Answer from the drawing. Dimensions are ordinates in mm from the lowest x, y and z of the part. A direction names the side the tool comes from. Coordinates: 2 decimals unless noted, no trailing zeros. Order: outer loops, then holes, each group sorted by start corner. A loop starts at its lowest first (then second) coordinate and runs counter-clockwise, first axis right, second up. Notation, with made-up numbers: (15, 7.25) -> (51, 7.25) arc R27 ccw to (51, 25.25) -> close; hole circle Ø5 at (19.25, -1). An arc over 180 degrees is marked (long way). Answer as a JSON object with one key per item and string values. Group by question number.
1) A tool of negligible diameter and unlimited length cuts with its end or side. For the marked faces 1 and 2, from which of +Z, -Z, +X, -X, +Y, -Y can it reach the whole face along a straight path? Write none if from no direction.
2) Given pin 1 (10.5 mm diameter, centred on x = 39.5, y = 15, fed in from -Z), flat-ended and moving along its own axis, determine where the tip first touches the part or whether it passes through.
3) Section C-C on z = 11.75 is taken. Determine the outline of the cut face in (x, y), and give its area (3 significant figures).
4) Determine the mould class of the marked faces 3, 4 and 5 for opening direction Y: released by +Y, released by -Y, zero draft, split by the parting line, or undercut.
5) Section A-A on y = 15 is taken. Count the separate pieces of the cut face and the enclosed holes in it, and give its area (3 significant figures).
6) Consider L1, parallel to Y at x = 8.5, z = 15; L2, parallel to Y at x = 42, z = 15; L3, parallel to X at y = 13.25, z = 8.5. Determine where each line is inside the solid, lowest interval first.
7) Section B-B on x = 8.5 is taken. Determine the outline of the cut face in (y, z).
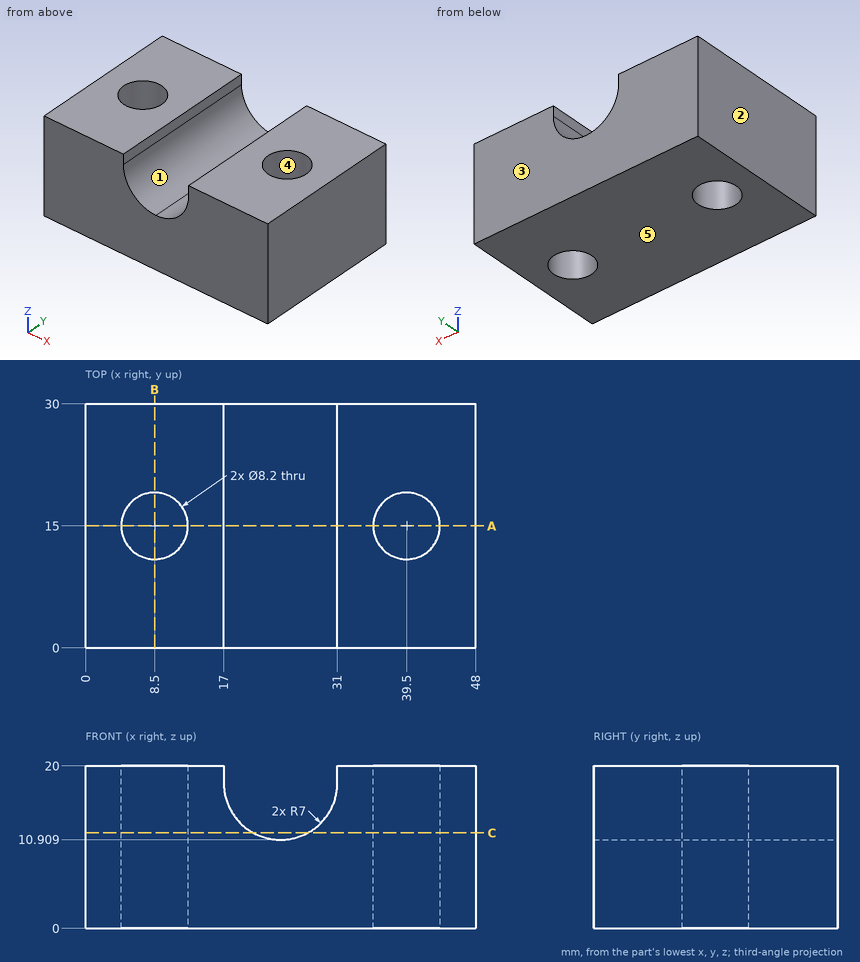
Worked answers:
{
 "1": {"face 1": "+Z, +Y, -Y", "face 2": "+Z, -Z, -X, +Y, -Y"},
 "2": {"pin 1": "stops at z = 0"},
 "3": {"outline": "(0, 0) -> (20.67, 0) -> (20.67, 30) -> (0, 30) -> close; (27.33, 0) -> (48, 0) -> (48, 30) -> (27.33, 30) -> close; hole circle Ø8.2 at (8.5, 15); hole circle Ø8.2 at (39.5, 15)", "area": "1,130 mm²"},
 "4": {"face 3": "released by +Y", "face 4": "undercut", "face 5": "zero draft"},
 "5": {"separate pieces": "3", "enclosed holes": "0", "area": "526 mm²"},
 "6": {"L1": "y = 0 to 10.9, 19.1 to 30", "L2": "y = 0 to 11.75, 18.25 to 30", "L3": "x = 0 to 4.79, 12.21 to 35.79, 43.21 to 48"},
 "7": {"outline": "(0, 0) -> (10.9, 0) -> (10.9, 20) -> (0, 20) -> close; (19.1, 0) -> (30, 0) -> (30, 20) -> (19.1, 20) -> close"}
}
